```python
from build123d import *

# Parameters (mm, degrees)
BOSS_EXTRUDE1_DEPTH   = 12.7
BOSS_EXTRUDE1_2_DEPTH = 12.7
SKETCH1_3_W           = 2.921
SKETCH1_3_H           = 5.588
BOSS_EXTRUDE2_DEPTH   = 6.35
SKETCH3_R             = 1.5875
CUT_EXTRUDE1_DEPTH    = 20.32
SKETCH4_W             = 7.9375
SKETCH4_H             = 6.35
CUT_EXTRUDE2_DEPTH    = 6.35


with BuildPart() as part:
    # Sketch1 → Boss-Extrude1 (new body)
    with BuildSketch(Plane.XY):
        Polygon((34.925, 12.7), (3.175, 12.7), (3.175, 13.6525), (0, 13.6525), (-3.175, 13.6525), (-3.175, 12.7), (-34.925, 12.7), (-34.925, 15.875), (34.925, 15.875), align=None)
    extrude(amount=-BOSS_EXTRUDE1_DEPTH)



with BuildPart() as body_2:
    # Sketch1 → Boss-Extrude1 2 (new body)
    with BuildSketch(Plane.XY):
        Polygon((-34.925, -12.7), (-3.175, -12.7), (-3.175, -13.6525), (0, -13.6525), (3.175, -13.6525), (3.175, -12.7), (34.925, -12.7), (34.925, -15.875), (-34.925, -15.875), align=None)
    extrude(amount=-BOSS_EXTRUDE1_2_DEPTH)


with BuildPart() as part_1:
    add(part.part)

    add(body_2.part)  # Boss-Extrude2 merges body 2
    # Sketch1_3 → Boss-Extrude2 (add)
    with BuildSketch(Plane.XY):
        Polygon((-34.925, -12.7), (-3.175, -12.7), (3.175, -12.7), (34.925, -12.7), (34.925, 12.7), (3.175, 12.7), (-3.175, 12.7), (-34.925, 12.7), align=None)
        with Locations((-15.1765, 0)):
            Rectangle(SKETCH1_3_W, SKETCH1_3_H, mode=Mode.SUBTRACT)
        Polygon((3.175, -6.604), (0, -6.604), (-3.175, -6.604), (-3.175, -2.794), (-7.366, -2.794), (-7.366, 2.794), (-3.175, 2.794), (-3.175, 6.604), (0, 6.604), (3.175, 6.604), (3.175, 2.794), (7.366, 2.794), (7.366, -2.794), (3.175, -2.794), align=None, mode=Mode.SUBTRACT)
        with Locations((15.1765, 0)):
            Rectangle(SKETCH1_3_W, SKETCH1_3_H, mode=Mode.SUBTRACT)
        Polygon((34.925, 12.7), (3.175, 12.7), (3.175, 13.6525), (0, 13.6525), (-3.175, 13.6525), (-3.175, 12.7), (-34.925, 12.7), (-34.925, 15.875), (34.925, 15.875), align=None)
        Polygon((-34.925, -12.7), (-3.175, -12.7), (-3.175, -13.6525), (0, -13.6525), (3.175, -13.6525), (3.175, -12.7), (34.925, -12.7), (34.925, -15.875), (-34.925, -15.875), align=None)
        Polygon((-3.175, 13.6525), (-3.175, 12.7), (3.175, 12.7), (3.175, 13.6525), (0, 13.6525), align=None)
        Polygon((3.175, -12.7), (-3.175, -12.7), (-3.175, -13.6525), (0, -13.6525), (3.175, -13.6525), align=None)
    extrude(amount=BOSS_EXTRUDE2_DEPTH)

    # Sketch3 → Cut-Extrude1 (cut)
    with BuildSketch(Plane(origin=(0, 15.875, 0), x_dir=(1, 0, 0), z_dir=(0, 1, 0))):
        with Locations((22.225, -3.175)):
            Circle(SKETCH3_R)
        with Locations((-22.225, -3.175)):
            Circle(SKETCH3_R)
    extrude(amount=-CUT_EXTRUDE1_DEPTH, mode=Mode.SUBTRACT)

    # Sketch4 → Cut-Extrude2 (cut)
    with BuildSketch(Plane.XY.offset(6.35)):
        with Locations((-22.225, 3.175)):
            Rectangle(SKETCH4_W, SKETCH4_H)
        with Locations((22.225, 3.175)):
            Rectangle(SKETCH4_W, SKETCH4_H)
    extrude(amount=-CUT_EXTRUDE2_DEPTH, mode=Mode.SUBTRACT)


solid = part_1.part
```
CAD build for the part. Positions are in the model's coordinates, mm. A direction names the side the tool comes from. Coordinates: 2 decimals unless noted, no trailing zeros. Order: outer loops, then holes, each group sorted by start corner. A loop starts at its lowest first (then second) coordinate and runs counter-clockwise, first axis right, second up. Notation, with made-up numbers: (43, -11) -> (75, -11) arc R20 cw to (75, 19) -> close; hole circle Ø6 at (66, 4.5). An arc over 180 degrees is marked (long way). Use one line per item in the form item = value. Start each with the question number.
1) Drop flat-ended pins along their axis: pin 1 (1 mm diameter, centred on x = 1, y = -9, fed in from -Z); pin 2 (1.9 mm diameter, centred on x = -22.225, z = 3.175, fed in from +Y) (3 decimals). Give the stop position or say it passes through.
2) Band-saw the part on C-C on z = -6.5. Give the cut face in (x, y) (1 decimal), then the cut area to 3 significant figures.
3) Band-saw the part on D-D on y = 5. Give the cut face in (x, z) (3 decimals).
4) Drill centre lines: L1, parallel to Y at x = 0, z = -8 (1 decimal); L2, parallel to X at y = -6, z = 4.75 (3 decimals); L3, parallel to Y at x = -6.5, z = 1.25 (3 decimals). Where is each one in solid material? Low to high. Write a range as [from, to].
5) Pull direction Z, two halves, no side cores. Call faces 1 (the cylindrical face through (20.64, -2.19, 3.11)), 2 (the flat face through (13.716, 0, 3)), 3 (the flat face through (0, 14, -12.7)): +Z half, -Z half, draft (parallel to the pull), parting line (faces both ways), or undercut.
6) Tool access for faces 4 (the flat face through (0, 15.875, -3)), 5 (the cylindrical face through (-20.759, -2.191, 3.783)), 6 (the flat face through (-5, 2.794, 3)): list every direction of +Z, -Z, +X, -X, +Y, -Y with a clear straight run to the whole face (end or side of a thin tool).
7) Band-saw the part on A-A on y = -5.5. Give the cut face in (x, z) (3 decimals), then the cut area to 3 significant figures.
Entries:
q1.pin_1 = 0
q1.pin_2 = -4.445
q2.outline = (-34.9, -15.9) -> (34.9, -15.9) -> (34.9, -12.7) -> (3.2, -12.7) -> (3.2, -13.7) -> (-3.2, -13.7) -> (-3.2, -12.7) -> (-34.9, -12.7) -> close; (-34.9, 12.7) -> (-3.2, 12.7) -> (-3.2, 13.7) -> (3.2, 13.7) -> (3.2, 12.7) -> (34.9, 12.7) -> (34.9, 15.9) -> (-34.9, 15.9) -> close
q2.area = 431 mm2
q3.outline = (-34.925, 0) -> (-26.194, 0) -> (-26.194, 6.35) -> (-34.925, 6.35) -> close; (-18.256, 0) -> (-3.175, 0) -> (-3.175, 6.35) -> (-18.256, 6.35) -> close; (3.175, 0) -> (18.256, 0) -> (18.256, 6.35) -> (3.175, 6.35) -> close; (26.194, 0) -> (34.925, 0) -> (34.925, 6.35) -> (26.194, 6.35) -> close
q4.L1 = [-15.9, -13.7], [13.7, 15.9]
q4.L2 = [-34.925, -3.175], [3.175, 34.925]
q4.L3 = [-15.875, -2.794], [2.794, 15.875]
q5.face_1 = undercut
q5.face_2 = draft
q5.face_3 = -Z half
q6.face_4 = +Z, -Z, +X, -X, +Y
q6.face_5 = +Y
q6.face_6 = +Z, -Z
q7.outline = (-34.925, 0) -> (-3.175, 0) -> (-3.175, 6.35) -> (-34.925, 6.35) -> close; (3.175, 0) -> (34.925, 0) -> (34.925, 6.35) -> (3.175, 6.35) -> close
q7.area = 403 mm2
